CAD build for the part. Positions are in the model's coordinates, mm. A direction names the side the tool comes from. Coordinates: 2 decimals unless noted, no trailing zeros. Loops run counter-clockwise (first coordinate to the right, second up) from the corner with the lowest first, then second, coordinate; pieces in that order, holes last.
1) Two-plate mould, pull along X, no slides. Class faces 4 (the flat face through (-3, 14, 1)), 5 (the flat face through (-1.5, -5, 0)), 6 (the flat face through (0, 0, 0)): +X half, -X half, draft (parallel to the pull), parting line (faces both ways), or undercut.
2) Saw through at D-D, the plane x = 3.25. Write the cut outline in (y, z), and give its area (3 significant figures).
3) Pin check, flat tips, straight feed: pin 1 Ø2 at (y, z) = (-7, 1.5) entering from +X; pin 2 Ø1 at (y, z) = (3, -4) entering from -X; pin 3 Ø2 at (y, z) = (9.5, -4) entering from +X. Stop position of each tip, or through.
4) Wall check: line 1 along X through (y, z) = (5.25, 0); line 2 along Z through (x, y) = (1.5, 0.25); line 3 along X through (y, z) = (4.5, 1.75). Give the ranges that are in metal, low to high.
5) Saw through at C-C, the plane y = 1. Write the cut outline in (x, z).
6) Which spindle directions (+Z, -Z, +X, -X, +Y, -Y) get a long thin tool onto all of the face, cutting with end or side? Do faces 1 (the flat face through (1.5, -5, 0)), 2 (the cylindrical face through (0.007, -9.787, -0.151)), 3 (the cylindrical face through (-2.53, 5.89, -3.29)). Say none if no direction does.
7) Saw through at B-B, the plane x = 2. Write the cut outline in (y, z), and give its area (3 significant figures).
8) Saw through at A-A, the plane z = 0. Write the cut outline in (x, y).
```python
from build123d import *

# Parameters (mm, degrees)
SKETCH1_R           = 4.15
SKETCH1_R_2         = 3
BOSS_EXTRUDE1_DEPTH = 14
BOSS_EXTRUDE2_START = -2
SKETCH1_2_R         = 4.15
SKETCH1_2_R_2       = 3
BOSS_EXTRUDE2_DEPTH = 2
BOSS_EXTRUDE3_DEPTH = 1.5
FILLET1_R           = 1


with BuildPart() as part:
    # Sketch1 → Boss-Extrude1 (new body)
    with BuildSketch(Plane(origin=(0, 0, 0), x_dir=(1, 0, 0), z_dir=(0, 1, 0))):
        with Locations(Location((0, 0, 0), (0, 0, 270))):
            Circle(SKETCH1_R)
        with Locations(Location((0, 0, 0), (0, 0, 270))):
            Circle(SKETCH1_R_2, mode=Mode.SUBTRACT)
    extrude(amount=BOSS_EXTRUDE1_DEPTH)

    # Sketch1<2> → Boss-Extrude2 (add)
    # profile 1 of 2: a face of its own
    with BuildSketch(Plane(origin=(0, 0, 0), x_dir=(1, 0, 0), z_dir=(0, 1, 0)).offset(BOSS_EXTRUDE2_START)):
        with Locations(Location((0, 0, 0), (0, 0, 270))):
            Circle(SKETCH1_2_R)
        with Locations(Location((0, 0, 0), (0, 0, 270))):
            Circle(SKETCH1_2_R_2, mode=Mode.SUBTRACT)
    # profile 2 of 2: a face of its own
    with BuildSketch(Plane(origin=(0, 0, 0), x_dir=(1, 0, 0), z_dir=(0, 1, 0)).offset(BOSS_EXTRUDE2_START)):
        with Locations(Location((0, 0, 0), (0, 0, 270))):
            Circle(SKETCH1_2_R_2)
    extrude(amount=BOSS_EXTRUDE2_DEPTH)

    # Sketch3 → Boss-Extrude3 (add, symmetric)
    with BuildSketch(Plane(origin=(0, 0, 0), x_dir=(0, 0, -1), z_dir=(1, 0, 0))):
        with BuildLine():
            Line((-4.15, -2), (4.15, -2))
            ThreePointArc((4.15, -2), (0, -9.788816953), (-4.15, -2))
        make_face()
    extrude(amount=BOSS_EXTRUDE3_DEPTH, both=True)

    # Fillet1
    # the kernel refuses this fillet: 1 mm, written as the material it takes off along each edge
    with BuildSketch(Plane(origin=(-1.5, -4.788816953, 0), x_dir=(0, 0.8881088245588202, -0.45963324046542875), z_dir=(0, 0.45963324046542875, 0.8881088245588202))) as fillet1_piece_1_section:
        with BuildLine():
            CenterArc((5 - FILLET1_R, -FILLET1_R), FILLET1_R, 0, 90)
            Line((5 - FILLET1_R, 0), (5, 0))
            Line((5, 0), (5, -FILLET1_R))
        make_face()
    fillet1_piece_1 = revolve(axis=Axis((-1.5, -4.788816953, 0), (-1, 0, 0)), revolution_arc=305.273112573, mode=Mode.PRIVATE)
    fillet1_piece_1 = split(fillet1_piece_1, bisect_by=Plane(origin=(-1.219469411, -2, 0), z_dir=(0, -1, 0)), keep=Keep.TOP, mode=Mode.PRIVATE)
    add(fillet1_piece_1, mode=Mode.SUBTRACT)
    with BuildSketch(Plane(origin=(1.5, -4.788816953, 0), x_dir=(0, 0.8881088245588202, -0.45963324046542875), z_dir=(0, 0.45963324046542875, 0.8881088245588202))) as fillet1_piece_2_section:
        with BuildLine():
            CenterArc((5 - FILLET1_R, FILLET1_R), FILLET1_R, 270, 90)
            Line((5 - FILLET1_R, 0), (5, 0))
            Line((5, 0), (5, FILLET1_R))
        make_face()
    fillet1_piece_2 = revolve(axis=Axis((1.5, -4.788816953, 0), (-1, 0, 0)), revolution_arc=305.273112573, mode=Mode.PRIVATE)
    fillet1_piece_2 = split(fillet1_piece_2, bisect_by=Plane(origin=(1.219469411, -2, 0), z_dir=(0, -1, 0)), keep=Keep.TOP, mode=Mode.PRIVATE)
    add(fillet1_piece_2, mode=Mode.SUBTRACT)


solid = part.part
```
Data:
1. face 4: draft
1. face 5: -X half
1. face 6: undercut
2. outline: (-2, -2.58) - (14, -2.58) - (14, 2.58) - (-2, 2.58) - close
2. area: 82.6 mm2
3. pin 1: stops at x = 1.5
3. pin 2: stops at x = -2.23
3. pin 3: stops at x = 2.87
4. line 1: x = -4.15 to -3, 3 to 4.15
4. line 2: z = -3.87 to -2.6, 2.6 to 3.87
4. line 3: x = -3.76 to -2.44, 2.44 to 3.76
5. outline: circle Ø8.3 at (0, 0); hole circle Ø6 at (0, 0)
6. face 1: +Z, -Z, +X, -Y
6. face 2: +X, -X
6. face 3: +Y
7. outline: (-2, -3.64) - (14, -3.64) - (14, -2.24) - (0, -2.24) - (0, 2.24) - (14, 2.24) - (14, 3.64) - (-2, 3.64) - close
7. area: 53.8 mm2
8. outline: (-4.15, -2) - (-1.5, -2) - (-1.5, -8.79) arc R1 ccw to (-0.5, -9.79) - (0.5, -9.79) arc R1 ccw to (1.5, -8.79) - (1.5, -2) - (4.15, -2) - (4.15, 14) - (3, 14) - (3, 0) - (-3, 0) - (-3, 14) - (-4.15, 14) - close
